Verification items for the finished model (mm, model axes). A direction names the side the tool comes from. Round coordinates to 2 decimals unless told otherwise and drop trailing zeros. Write each loop counter-clockwise with the first axis right and the second up, starting at its lowest first coordinate (ties: lowest second). Pieces come first, ordered by that corner, then holes.
from build123d import *

# Parameters (mm, degrees)
SKETCH_W        = 30
SKETCH_H        = 9
PAD_DEPTH       = 5.5
SKETCH001_R     = 0.4
POCKET_DEPTH    = 10
SKETCH002_W     = 20.2
SKETCH002_H     = 2.5
POCKET001_DEPTH = 1
FILLET_R        = 0.5
FILLET001_R     = 0.5
SKETCH003_W     = 1.5
SKETCH003_H     = 0.5
PAD001_DEPTH    = 4
SKETCH004_R     = 0.6
PAD002_DEPTH    = 4.5


with BuildPart() as part:
    # Sketch → Pad (new body)
    with BuildSketch(Plane.XY):
        with Locations((15, 4.5)):
            Rectangle(SKETCH_W, SKETCH_H)
    extrude(amount=PAD_DEPTH)

    # Sketch001 → Pocket (cut)
    with BuildSketch(Plane.XY.offset(5.5)):
        with Locations((2, 4.5)):
            Circle(SKETCH001_R)
        with Locations((28, 4.5)):
            Circle(SKETCH001_R)
    extrude(amount=-POCKET_DEPTH, mode=Mode.SUBTRACT)

    # Sketch002 → Pocket001 (cut)
    with BuildSketch(Plane.XY.offset(5.5)):
        with Locations((15, 4.5)):
            Rectangle(SKETCH002_W, SKETCH002_H)
    extrude(amount=-POCKET001_DEPTH, mode=Mode.SUBTRACT)

    # Fillet
    fillet_edges = [part.edges().sort_by_distance(p)[0] for p in [
        (0, 4.5, 5.5),
    ]]
    fillet(fillet_edges, radius=FILLET_R)

    # Fillet001
    fillet001_edges = [part.edges().sort_by_distance(p)[0] for p in [
        (30, 4.5, 5.5),
    ]]
    fillet(fillet001_edges, radius=FILLET001_R)

    # Sketch003 → Pad001 (new body)
    with BuildSketch(Plane(origin=(0, 0, 0), x_dir=(1, 0, 0), z_dir=(0, 0, -1))):
        with Locations((6.1, -0.25)):
            Rectangle(SKETCH003_W, SKETCH003_H)
        with Locations((23.9, -0.25)):
            Rectangle(SKETCH003_W, SKETCH003_H)
        with Locations((4.9, -8.75)):
            Rectangle(SKETCH003_W, SKETCH003_H)
        with Locations((25.1, -8.75)):
            Rectangle(SKETCH003_W, SKETCH003_H)
    extrude(amount=PAD001_DEPTH)

    # Sketch004 → Pad002 (new body)
    with BuildSketch(Plane(origin=(0, 0, 0), x_dir=(1, 0, 0), z_dir=(0, 0, -1))):
        with Locations((29.25, -6.25)):
            Circle(SKETCH004_R)
        with Locations((0.75, -6.25)):
            Circle(SKETCH004_R)
        with Locations((29.25, -2.75)):
            Circle(SKETCH004_R)
    extrude(amount=PAD002_DEPTH)


solid = part.part
Q1. Sectioned sample at B-B (x = 2). Enter the section's corners in (y, z), plus the area to 3 significant figures.
Recorded:
outline: (0, 0) - (4.1, 0) - (4.1, 5.5) - (0, 5.5) - close; (4.9, 0) - (9, 0) - (9, 5.5) - (4.9, 5.5) - close
area: 45.1 mm2
Q2. Depth check by flat-ended pin: P1, Ø0.6, axis at y = 9, z = -1, coming from the -X side; P2, Ø1.5, axis at y = 2.5, z = -3.5, coming from the +X side; P3, Ø4.5, axis at x = 12, y = 2.5, coming from the -Z side. Enter the tip coordinate at first touch or a pass-through.
Recorded:
P1: stops at x = 4.15
P2: stops at x = 29.85
P3: stops at z = 0
Q3. Tool access check on faces 1 (the flat face through (24, 0.5, -2)), 2 (the flat face through (15, 5.75, 5)), 3 (the flat face through (1, 6, -4.5)), 4 (the cylindrical face through (29.804, 2.98, -2.218)). Record the directions out of +Z, -Z, +X, -X, +Y, -Y that give a thin tool (end or side, any length) a straight path to the whole face; none if there is none.
Recorded:
face 1: -Z, +X, -X
face 2: +Z
face 3: -Z, +X, -X, +Y, -Y
face 4: -Z
Q4. Sectioned sample at A-A (y = 4.5). Enter the section's corners in (x, z).
Recorded:
outline: (0, 0) - (1.6, 0) - (1.6, 5.5) - (0.5, 5.5) arc R0.5 ccw to (0, 5) - close; (2.4, 0) - (27.6, 0) - (27.6, 5.5) - (25.1, 5.5) - (25.1, 4.5) - (4.9, 4.5) - (4.9, 5.5) - (2.4, 5.5) - close; (28.4, 0) - (30, 0) - (30, 5) arc R0.5 ccw to (29.5, 5.5) - (28.4, 5.5) - close
Q5. Sectioned sample at D-D (y = 2.75). Enter the section's corners in (x, z), plus the area to 3 significant figures.
Recorded:
outline: (0, 0) - (28.65, 0) - (28.65, -4.5) - (29.85, -4.5) - (29.85, 0) - (30, 0) - (30, 5) arc R0.5 ccw to (29.5, 5.5) - (0.5, 5.5) arc R0.5 ccw to (0, 5) - close
area: 170 mm2
Q6. Sectioned sample at C-C (x = 17.75). Enter the section's corners in (y, z).
Recorded:
outline: (0, 0) - (9, 0) - (9, 5.5) - (5.75, 5.5) - (5.75, 4.5) - (3.25, 4.5) - (3.25, 5.5) - (0, 5.5) - close
Q7. Material ranges on line 1 along X through (y, z) = (4.75, 2.25); line 2 along Y through (x, z) = (2, 3.95); line 3 along Y through (x, z) = (28.75, -2.5), recorded low to high.
Recorded:
line 1: x = 0 to 1.69, 2.31 to 27.69, 28.31 to 30
line 2: y = 0 to 4.1, 4.9 to 9
line 3: y = 2.42 to 3.08, 5.92 to 6.58
